from build123d import *

# Parameters (mm, degrees)
SKETCH_2_R            = 1.425
EXTRUDE_1_DEPTH       = 2
SKETCH_2_3_R          = 1.425
EXTRUDE_2_DEPTH       = 2
EXTRUDE_START         = -1
EXTRUDE_3_DEPTH       = 1
EXTRUDE_4_DEPTH       = 1
SKETCH_2_6_W          = 8.1
SKETCH_2_6_H          = 3
EXTRUDE_5_DEPTH       = 3.6
EXTRUDE_6_DEPTH       = 15.2
EXTRUDE_6_DEPTH_BACK  = 1
SKETCH_2_7_R          = 1.425
SKETCH_2_8_W          = 29.4
SKETCH_2_8_H          = 25
EXTRUDE_7_DEPTH       = 1
SKETCH_2_9_W          = 29.4
SKETCH_2_9_H          = 16
EXTRUDE_8_DEPTH       = 1
SKETCH_2_10_W         = 29.4
SKETCH_2_10_H         = 16
EXTRUDE_9_DEPTH       = 2
SKETCH_2_11_W         = 8.1
SKETCH_2_11_H         = 3
SKETCH_2_11_R         = 1.425
EXTRUDE_10_DEPTH      = 1
EXTRUDE_12_DEPTH      = 16.9
EXTRUDE_12_DEPTH_BACK = 1
SKETCH_2_24_W         = 1
SKETCH_2_24_H         = 1
EXTRUDE_13_DEPTH      = 16.9
SKETCH_2_25_W         = 13.1
SKETCH_2_25_H         = 1
EXTRUDE_14_DEPTH      = 15.2
SKETCH_2_26_W         = 8.1
SKETCH_2_26_H         = 1
EXTRUDE_15_DEPTH      = 3.6
SKETCH_2_28_W         = 1
SKETCH_2_28_H         = 1
SKETCH_2_28_W_2       = 13.1
SKETCH_2_28_W_3       = 8.1
EXTRUDE_16_DEPTH      = 1
FILLET_1_R            = 2
SKETCH_4_R            = 2.15
SKETCH_4_R_2          = 1.425
CUT_EXTRUDE_1_DEPTH   = 2.1


# Read off the part's stored shape, not the designer's step: the extrude step
with BuildPart() as part:
    # Sketch 2 → Extrude 1 (new body)
    with BuildSketch(Plane.XY):
        Polygon((-31.74588875, 30.116039863), (-37.24588875, 30.116039863), (-37.69588875, 30.116039863), (-37.69588875, 24.616039863), (-37.24588875, 24.616039863), (-31.74588875, 24.616039863), align=None)
        with Locations((-34.49588875, 27.616039863)):
            Circle(SKETCH_2_R, mode=Mode.SUBTRACT)
    extrude(amount=EXTRUDE_1_DEPTH)



with BuildPart() as body_2:
    # Sketch 2_3 → Extrude 2 (new body)
    with BuildSketch(Plane.XY):
        Polygon((-8.74588875, 30.116039863), (-14.24588875, 30.116039863), (-14.24588875, 24.616039863), (-8.74588875, 24.616039863), (-8.29588875, 24.616039863), (-8.29588875, 30.116039863), align=None)
        with Locations((-11.49588875, 27.616039863)):
            Circle(SKETCH_2_3_R, mode=Mode.SUBTRACT)
    extrude(amount=EXTRUDE_2_DEPTH)


with BuildPart() as body_3:
    # Extrude 3 outline → Extrude 3 (new body)
    with BuildSketch(Plane.XY.offset(EXTRUDE_START)):
        Polygon((-37.69588875, 24.616039863), (-37.69588875, 11.116039863), (-22.99588875, 11.116039863), (-22.99588875, 30.116039863), (-31.74588875, 30.116039863), (-31.74588875, 24.616039863), align=None)
    extrude(amount=EXTRUDE_3_DEPTH)

    # Sketch 2_5 → Extrude 4 (add)
    with BuildSketch(Plane.XY):
        Polygon((-22.99588875, 30.116039863), (-22.99588875, 28.589280798), (-22.99588875, 11.116039863), (-8.29588875, 11.116039863), (-8.29588875, 24.616039863), (-8.74588875, 24.616039863), (-14.24588875, 24.616039863), (-14.24588875, 30.116039863), (-14.89588875, 30.116039863), align=None)
    extrude(amount=-EXTRUDE_4_DEPTH)

    # Sketch 2_7 → Extrude 6 (add, two sides: drawn at the far end of the back side and taken through both)
    with BuildSketch(Plane.XY.offset(-EXTRUDE_6_DEPTH_BACK)):
        Polygon((-31.74588875, 30.116039863), (-31.09588875, 30.116039863), (-31.09588875, 33.116039863), (-44.19588875, 33.116039863), (-44.19588875, 11.116039863), (-44.19588875, -29.883960137), (-44.19588875, -39.883960137), (-1.79588875, -39.883960137), (-1.79588875, -29.883960137), (-1.79588875, 11.116039863), (-1.79588875, 33.116039863), (-14.89588875, 33.116039863), (-14.89588875, 30.116039863), (-14.24588875, 30.116039863), (-8.74588875, 30.116039863), (-8.29588875, 30.116039863), (-8.29588875, 24.616039863), (-8.29588875, 11.116039863), (-8.29588875, -4.883960137), (-8.29588875, -29.883960137), (-37.69588875, -29.883960137), (-37.69588875, -4.883960137), (-37.69588875, 11.116039863), (-37.69588875, 24.616039863), (-37.69588875, 30.116039863), (-37.24588875, 30.116039863), align=None)
        with Locations(Location((-41.39588875, -37.083960137, 0), (0, 0, 180))):
            Circle(SKETCH_2_7_R, mode=Mode.SUBTRACT)
        with Locations(Location((-4.59588875, -37.083960137, 0), (0, 0, 180))):
            Circle(SKETCH_2_7_R, mode=Mode.SUBTRACT)
        with Locations(Location((-41.39588875, 7.716039863, 0), (0, 0, 180))):
            Circle(SKETCH_2_7_R, mode=Mode.SUBTRACT)
        with Locations(Location((-41.39588875, 29.316039863, 0), (0, 0, 180))):
            Circle(SKETCH_2_7_R, mode=Mode.SUBTRACT)
        with Locations(Location((-4.59588875, 7.716039863, 0), (0, 0, 180))):
            Circle(SKETCH_2_7_R, mode=Mode.SUBTRACT)
        with Locations(Location((-4.59588875, 29.316039863, 0), (0, 0, 180))):
            Circle(SKETCH_2_7_R, mode=Mode.SUBTRACT)
    extrude(amount=EXTRUDE_6_DEPTH + EXTRUDE_6_DEPTH_BACK)

    # Sketch 2_8 → Extrude 7 (add)
    with BuildSketch(Plane.XY):
        with Locations((-22.99588875, -17.383960137)):
            Rectangle(SKETCH_2_8_W, SKETCH_2_8_H)
    extrude(amount=-EXTRUDE_7_DEPTH)

    # Sketch 2_9 → Extrude 8 (add)
    with BuildSketch(Plane.XY):
        with Locations((-22.99588875, 3.116039863)):
            Rectangle(SKETCH_2_9_W, SKETCH_2_9_H)
    extrude(amount=-EXTRUDE_8_DEPTH)

    # Sketch 2_10 → Extrude 9 (add)
    with BuildSketch(Plane.XY):
        with Locations((-22.99588875, 3.116039863)):
            Rectangle(SKETCH_2_10_W, SKETCH_2_10_H)
    extrude(amount=EXTRUDE_9_DEPTH)


with BuildPart() as body_4:
    # Sketch 2_6 → Extrude 5 (new body)
    with BuildSketch(Plane.XY):
        with Locations((-27.04588875, 31.616039863)):
            Rectangle(SKETCH_2_6_W, SKETCH_2_6_H)
        with Locations((-18.94588875, 31.616039863)):
            Rectangle(SKETCH_2_6_W, SKETCH_2_6_H)
    extrude(amount=EXTRUDE_5_DEPTH)


with BuildPart() as part_1:
    add(part.part)

    add(body_2.part)  # Extrude 10 merges body 2

    add(body_3.part)  # Extrude 10 merges body 3

    add(body_4.part)  # Extrude 10 merges body 4
    # Sketch 2_11 → Extrude 10 (add)
    # profile 1 of 4: a face of its own
    with BuildSketch(Plane.XY.offset(EXTRUDE_START)):
        with Locations((-18.94588875, 31.616039863)):
            Rectangle(SKETCH_2_11_W, SKETCH_2_11_H)
    # profile 2 of 4: a face of its own
    with BuildSketch(Plane.XY.offset(EXTRUDE_START)):
        with Locations((-27.04588875, 31.616039863)):
            Rectangle(SKETCH_2_11_W, SKETCH_2_11_H)
    # profile 3 of 4: a face of its own
    with BuildSketch(Plane.XY.offset(EXTRUDE_START)):
        Polygon((-8.74588875, 30.116039863), (-14.24588875, 30.116039863), (-14.24588875, 24.616039863), (-8.74588875, 24.616039863), (-8.29588875, 24.616039863), (-8.29588875, 30.116039863), align=None)
        with Locations((-11.49588875, 27.616039863)):
            Circle(SKETCH_2_11_R, mode=Mode.SUBTRACT)
    # profile 4 of 4: a face of its own
    with BuildSketch(Plane.XY.offset(EXTRUDE_START)):
        Polygon((-31.74588875, 24.616039863), (-31.74588875, 30.116039863), (-37.24588875, 30.116039863), (-37.69588875, 30.116039863), (-37.69588875, 24.616039863), (-37.24588875, 24.616039863), align=None)
        with Locations((-34.49588875, 27.616039863)):
            Circle(SKETCH_2_11_R, mode=Mode.SUBTRACT)
    extrude(amount=EXTRUDE_10_DEPTH)

    # Sketch 2_22 → Extrude 12 (add, two sides: drawn at the far end of the back side and taken through both)
    with BuildSketch(Plane.XY.offset(-EXTRUDE_12_DEPTH_BACK)):
        Polygon((-44.19588875, 11.116039863), (-44.19588875, 33.116039863), (-45.19588875, 33.116039863), (-45.19588875, -40.883960137), (-44.19588875, -40.883960137), (-0.79588875, -40.883960137), (-0.79588875, 33.116039863), (-1.79588875, 33.116039863), (-1.79588875, 11.116039863), (-1.79588875, -29.883960137), (-1.79588875, -39.883960137), (-44.19588875, -39.883960137), (-44.19588875, -29.883960137), align=None)
    extrude(amount=EXTRUDE_12_DEPTH + EXTRUDE_12_DEPTH_BACK)

    # Sketch 2_24 → Extrude 13 (add)
    with BuildSketch(Plane.XY):
        with Locations((-44.69588875, 33.616039863)):
            Rectangle(SKETCH_2_24_W, SKETCH_2_24_H)
        with Locations((-1.29588875, 33.616039863)):
            Rectangle(SKETCH_2_24_W, SKETCH_2_24_H)
    extrude(amount=EXTRUDE_13_DEPTH)

    # Sketch 2_25 → Extrude 14 (add)
    with BuildSketch(Plane.XY):
        with Locations((-37.64588875, 33.616039863)):
            Rectangle(SKETCH_2_25_W, SKETCH_2_25_H)
        with Locations((-8.34588875, 33.616039863)):
            Rectangle(SKETCH_2_25_W, SKETCH_2_25_H)
    extrude(amount=EXTRUDE_14_DEPTH)

    # Sketch 2_26 → Extrude 15 (add)
    with BuildSketch(Plane.XY):
        with Locations((-27.04588875, 33.616039863)):
            Rectangle(SKETCH_2_26_W, SKETCH_2_26_H)
        with Locations((-18.94588875, 33.616039863)):
            Rectangle(SKETCH_2_26_W, SKETCH_2_26_H)
    extrude(amount=EXTRUDE_15_DEPTH)

    # Sketch 2_28 → Extrude 16 (add)
    with BuildSketch(Plane.XY):
        with Locations((-1.29588875, 33.616039863)):
            Rectangle(SKETCH_2_28_W, SKETCH_2_28_H)
        with Locations((-8.34588875, 33.616039863)):
            Rectangle(SKETCH_2_28_W_2, SKETCH_2_28_H)
        with Locations((-18.94588875, 33.616039863)):
            Rectangle(SKETCH_2_28_W_3, SKETCH_2_28_H)
        with Locations((-27.04588875, 33.616039863)):
            Rectangle(SKETCH_2_28_W_3, SKETCH_2_28_H)
        with Locations((-37.64588875, 33.616039863)):
            Rectangle(SKETCH_2_28_W_2, SKETCH_2_28_H)
        with Locations((-44.69588875, 33.616039863)):
            Rectangle(SKETCH_2_28_W, SKETCH_2_28_H)
    extrude(amount=-EXTRUDE_16_DEPTH)

    # Fillet 1
    fillet_1_edges = [part_1.edges().sort_by_distance(p)[0] for p in [
        (-0.79588875, -40.883960137, 7.95),
        (-45.19588875, -40.883960137, 7.95),
        (-0.79588875, 34.116039863, 7.95),
        (-45.19588875, 34.116039863, 7.95),
    ]]
    fillet(fillet_1_edges, radius=FILLET_1_R)

    # Sketch 4 → Cut-Extrude 1 (cut)
    # profile 1 of 6: a face of its own
    with BuildSketch(Plane(origin=(0, 0, -1), x_dir=(-1, 0, 0), z_dir=(0, 0, -1))):
        with Locations((4.59588875, 7.716039863)):
            Circle(SKETCH_4_R)
        with Locations((4.59588875, 7.716039863)):
            Circle(SKETCH_4_R_2, mode=Mode.SUBTRACT)
    # profile 2 of 6: a face of its own
    with BuildSketch(Plane(origin=(0, 0, -1), x_dir=(-1, 0, 0), z_dir=(0, 0, -1))):
        with Locations((4.59588875, 29.316039863)):
            Circle(SKETCH_4_R)
        with Locations((4.59588875, 29.316039863)):
            Circle(SKETCH_4_R_2, mode=Mode.SUBTRACT)
    # profile 3 of 6: a face of its own
    with BuildSketch(Plane(origin=(0, 0, -1), x_dir=(-1, 0, 0), z_dir=(0, 0, -1))):
        with Locations((41.39588875, 29.316039863)):
            Circle(SKETCH_4_R)
        with Locations((41.39588875, 29.316039863)):
            Circle(SKETCH_4_R_2, mode=Mode.SUBTRACT)
    # profile 4 of 6: a face of its own
    with BuildSketch(Plane(origin=(0, 0, -1), x_dir=(-1, 0, 0), z_dir=(0, 0, -1))):
        with Locations((41.39588875, 7.716039863)):
            Circle(SKETCH_4_R)
        with Locations((41.39588875, 7.716039863)):
            Circle(SKETCH_4_R_2, mode=Mode.SUBTRACT)
    # profile 5 of 6: a face of its own
    with BuildSketch(Plane(origin=(0, 0, -1), x_dir=(-1, 0, 0), z_dir=(0, 0, -1))):
        with Locations((4.59588875, -37.083960137)):
            Circle(SKETCH_4_R)
        with Locations((4.59588875, -37.083960137)):
            Circle(SKETCH_4_R_2, mode=Mode.SUBTRACT)
    # profile 6 of 6: a face of its own
    with BuildSketch(Plane(origin=(0, 0, -1), x_dir=(-1, 0, 0), z_dir=(0, 0, -1))):
        with Locations((41.39588875, -37.083960137)):
            Circle(SKETCH_4_R)
        with Locations((41.39588875, -37.083960137)):
            Circle(SKETCH_4_R_2, mode=Mode.SUBTRACT)
    extrude(amount=-CUT_EXTRUDE_1_DEPTH, mode=Mode.SUBTRACT)


solid = part_1.part
Design review of the part built by this model. Coordinates are the model's own, in mm. A direction names the side the tool comes from. Give positions to 0.01 mm unless a question says otherwise; leave off trailing zeros. Write each loop counter-clockwise with the first axis right and the second up, starting at its lowest first coordinate (ties: lowest second). Pieces come first, ordered by that corner, then holes. Notation, with made-up numbers: M -6.75,44.5 L 6.25,44.5 A22 ccw 6.25,74.5 Z; hole C -12.75,46 d5. An arc over 180 degrees is marked long. Return JSON: item names as keys, results as strings. Group by question number.
Item 1: Tool access review of faces 5 (the flat face through (-23, 34.116, 2)), 6 (the cylindrical face through (-11.68, 29.03, 0.48)), 7 (the flat face through (-23, 11.116, 1)), 8 (the cylindrical face through (-5.75, 9.53, 0.04)), 9 (the flat face through (-23, 32, 3.6)): name each direction out of +Z, -Z, +X, -X, +Y, -Y from which nothing blocks a thin tool from reaching the whole face with its end or side.
Item 2: Clearance check with flat-ended pins moving along their axes: pin 1 Ø20 at (x, y) = (-24.5, -16.5) entering from +Z; pin 2 Ø3.5 at (x, y) = (-4, 29.5) entering from -Z; pin 3 Ø4.5 at (x, y) = (-34.5, 27.62) entering from +Z; pin 4 Ø12 at (x, y) = (-37, 13) entering from +Z. State where each tip first meets the part, or that it passes through.
Item 3: Take a section at A-A (y = 17). Give the boundary of the cut face in (x, z), plus the area to 3 significant figures.
Item 4: Take a section at D-D (y = -31). Give the boundary of the cut face in (x, z).
Item 5: The part is to be moulded in two halves that separate along Y. For faces 1 (the flat face through (-5, 31, 1.1)), 2 (the flat face through (-39, -8, 15.2)), 3 (the flat face through (-23, -40.884, 8)), 4 (the cylindrical face through (-40.35, -38.05, 8.05)), say which applies: pulls with the +Y half, pulls with the -Y half, needs draft (parallel to the pull), parting line crosses it, or undercut.
Item 6: Take a section at C-C (z = 5). Give the boundary of the cut face in (x, y) (3 decimals).
Item 7: Take a section at B-B (x = -17). Give the boundary of the cut face in (y, z).
Item 8: Wall thickness on line 1 along Y through (x, z) = (-22.5, 0.5); line 2 along Y through (x, z) = (-36, 3); line 3 along Y through (x, z) = (-41, 10.75): over which ranges is each line inside the solid? List them lowest first.
Return value:
{
 "1": {"face 5": "+Z, -Z, +X, -X, +Y", "face 6": "+Z, -Z", "face 7": "+Z", "face 8": "-Z", "face 9": "+Z, +Y"},
 "2": {"pin 1": "stops at z = 0", "pin 2": "stops at z = -1", "pin 3": "stops at z = 2", "pin 4": "stops at z = 15.2"},
 "3": {"outline": "M -45.2,-1 L -0.8,-1 L -0.8,16.9 L -1.8,16.9 L -1.8,15.2 L -8.3,15.2 L -8.3,0 L -37.7,0 L -37.7,15.2 L -44.2,15.2 L -44.2,16.9 L -45.2,16.9 Z", "area": "276 mm2"},
 "4": {"outline": "M -45.2,-1 L -0.8,-1 L -0.8,16.9 L -1.8,16.9 L -1.8,15.2 L -44.2,15.2 L -44.2,16.9 L -45.2,16.9 Z"},
 "5": {"face 1": "undercut", "face 2": "needs draft", "face 3": "pulls with the -Y half", "face 4": "undercut"},
 "6": {"outline": "M -45.196,-38.884 A2 ccw -43.196,-40.884 L -2.796,-40.884 A2 ccw -0.796,-38.884 L -0.796,32.116 A2 ccw -2.796,34.116 L -14.896,34.116 L -14.896,30.116 L -8.296,30.116 L -8.296,-29.884 L -37.696,-29.884 L -37.696,30.116 L -31.096,30.116 L -31.096,34.116 L -43.196,34.116 A2 ccw -45.196,32.116 Z; hole C -41.396,-37.084 d2.85; hole C -41.396,7.716 d2.85; hole C -41.396,29.316 d2.85; hole C -4.596,-37.084 d2.85; hole C -4.596,7.716 d2.85; hole C -4.596,29.316 d2.85"},
 "7": {"outline": "M -40.88,-1 L 34.12,-1 L 34.12,3.6 L 30.12,3.6 L 30.12,0 L 11.12,0 L 11.12,2 L -4.88,2 L -4.88,0 L -29.88,0 L -29.88,15.2 L -39.88,15.2 L -39.88,16.9 L -40.88,16.9 Z"},
 "8": {"line 1": "y = -40.88 to -29.88, -4.88 to 11.12, 30.12 to 34.12", "line 2": "y = -40.88 to -29.88, 30.12 to 34.12", "line 3": "y = -40.88 to -38.45, -35.72 to 6.35, 9.08 to 27.95, 30.68 to 34.12"}
}
